Answer from the drawing. Dimensions are ordinates in mm from the lowest x, y and z of the part. Coordinates: 2 decimals unless noted, no trailing zeros. Order: outer loops, then holes, each group sorted by start corner. A loop starts at its lowest first (then second) coordinate and runs counter-clockwise, first axis right, second up. Notation, with made-up numbers: (-33.75, 50) - (-5.75, 50) arc R24 cw to (-5.75, 61) - close; hole circle Ø9 at (-37, 4.25). An arc over 180 degrees is marked (long way). Use CSV: the item, a comma, the result in double quotes. Start each with the question number.
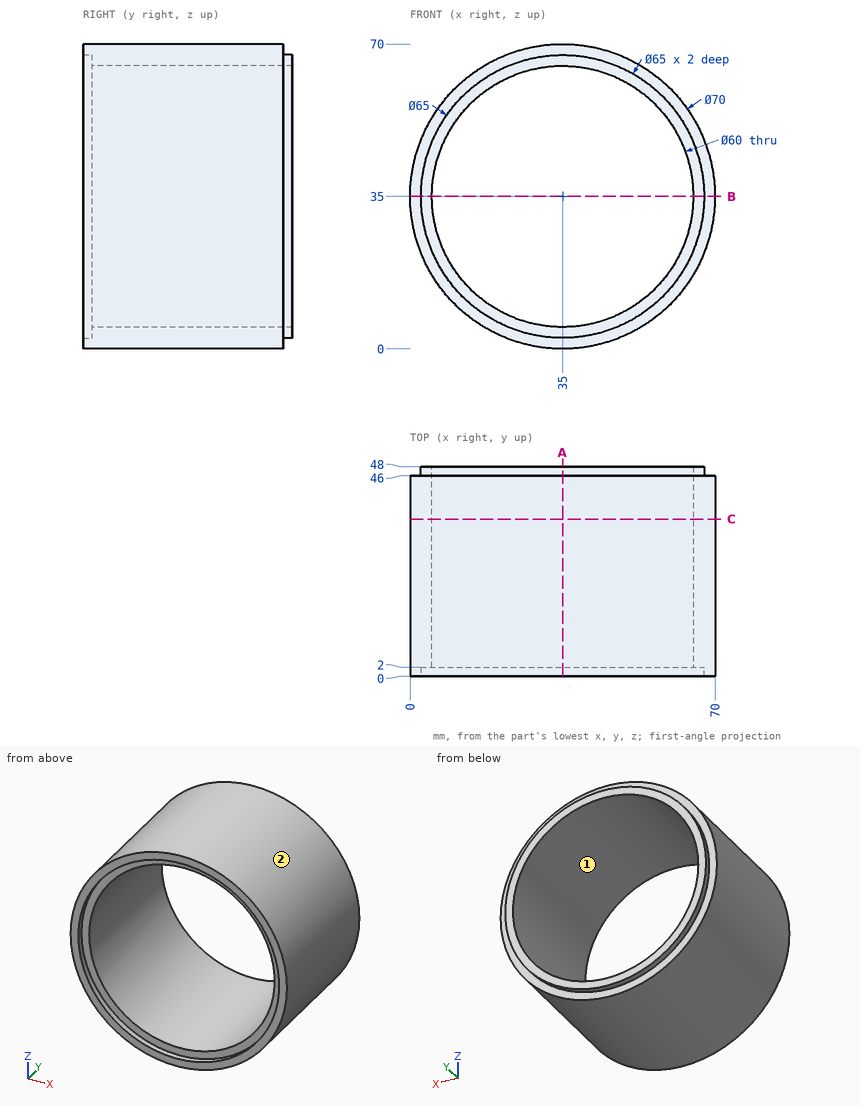
1) The part is cut by section A-A on x = 35. Determine the outline of the cut face in (y, z).
2) Flat-ended cylindrical pins translate along their axes: P1, Ø1.5, axis at x = 20, y = 23, coming from the -Z side; P2, Ø6, axis at y = 21.5, z = 47.5, coming from the +X side; P3, Ø12, axis at x = 30.5, y = 7.5, coming from the +Z side; P4, Ø5, axis at y = 20.5, z = 36, coming from the -X side. Find the tip coordinate at first contact, or state that the pin passes through.
3) For a pull along X with two mould halves and no side action, classify the marked faces 1 and 2 as +X half, -X half, draft (parallel to the pull), parting line (faces both ways), or undercut.
4) Straight lines are drawn through the part: line 1 (Z direction, x = 35, y = 24); line 2 (X direction, y = 28.5, z = 50); line 3 (Z direction, x = 44, y = 42). For each, find the intervals that lie inside material, in ascending order. Write a range as [from, to].
5) The part is cut by section B-B on z = 35. Determine the outline of the cut face in (x, y).
6) The part is cut by section C-C on y = 36. Determine the outline of the cut face in (x, z), plus the area to 3 significant figures.
Answer key:
1,outline,"(0, 0) - (46, 0) - (46, 2.5) - (48, 2.5) - (48, 5) - (2, 5) - (2, 2.5) - (0, 2.5) - close; (0, 67.5) - (2, 67.5) - (2, 65) - (48, 65) - (48, 67.5) - (46, 67.5) - (46, 70) - (0, 70) - close"
2,P1,"z = 3.03"
2,P2,"x = 68.69"
2,P3,"z = 70"
2,P4,"x = 0"
3,face 1,"undercut"
3,face 2,"parting line"
4,line 1,"[0, 5], [65, 70]"
4,line 2,"[3.38, 9.02], [60.98, 66.62]"
4,line 3,"[1.18, 6.38], [63.62, 68.82]"
5,outline,"(0, 0) - (2.5, 0) - (2.5, 2) - (5, 2) - (5, 48) - (2.5, 48) - (2.5, 46) - (0, 46) - close; (65, 2) - (67.5, 2) - (67.5, 0) - (70, 0) - (70, 46) - (67.5, 46) - (67.5, 48) - (65, 48) - close"
6,outline,"circle Ø70 at (35, 35); hole circle Ø60 at (35, 35)"
6,area,"1,020 mm^2"
